Work out the finished part from the listing and answer in its coordinate system (mm). A direction names the side the tool comes from. Give positions to 0.01 mm unless a question says otherwise; leave off trailing zeros. Loops run counter-clockwise (first coordinate to the right, second up) from the corner with the lowest first, then second, coordinate; pieces in that order, holes last. Notation, with made-up numbers: (-17.75, 37.5) - (25.25, 37.5) arc R28 ccw to (25.25, 60.5) - close; hole circle Ø2 at (-1.5, -5). An arc over 180 degrees is marked (long way). One line per item, written item: value.
from build123d import *

# Parameters (mm, degrees)
SKETCH1_R           = 1.45
SKETCH1_W           = 3.4
SKETCH1_H           = 6.165
BOSS_EXTRUDE1_DEPTH = 6


with BuildPart() as part:
    # Sketch1 → Boss-Extrude1 (new body)
    with BuildSketch(Plane.XY):
        with BuildLine():
            Line((589.771388, 466.232899), (612.771388, 466.232899))
            ThreePointArc((612.771388, 466.232899), (618.521388, 460.482899), (612.771388, 454.732899))
            Line((612.771388, 454.732899), (589.771388, 454.732899))
            Line((589.771388, 454.732899), (586.771388, 454.732899))
            ThreePointArc((586.771388, 454.732899), (581.021388, 460.482899), (586.771388, 466.232899))
            Line((586.771388, 466.232899), (589.771388, 466.232899))
        make_face()
        with Locations((589.771388, 460.482899)):
            Circle(SKETCH1_R, mode=Mode.SUBTRACT)
        with Locations((612.771388, 460.482899)):
            Circle(SKETCH1_R, mode=Mode.SUBTRACT)
        with Locations((595.021388, 460.482899)):
            Rectangle(SKETCH1_W, SKETCH1_H, mode=Mode.SUBTRACT)
    extrude(amount=BOSS_EXTRUDE1_DEPTH)


solid = part.part
1. The mould has two halves that part along Y. Classify faces 3 (the flat face through (593.321, 460, 3)), 4 (the flat face through (600, 454.733, 3)), 5 (the flat face through (600, 461, 6)): released by +Y, released by -Y, zero draft, split by the parting line, or undercut.
Output:
face 3: undercut
face 4: released by -Y
face 5: zero draft
2. Section B-B (y = 461.25) is taken. Write down the section's boundary in (x, z).
Output:
outline: (581.07, 0) - (588.54, 0) - (588.54, 6) - (581.07, 6) - close; (591, 0) - (593.32, 0) - (593.32, 6) - (591, 6) - close; (596.72, 0) - (611.54, 0) - (611.54, 6) - (596.72, 6) - close; (614, 0) - (618.47, 0) - (618.47, 6) - (614, 6) - close
3. Section A-A (x = 595.5) is taken. Write down the section's boundary in (y, z), and give its area (3 significant figures).
Output:
outline: (454.73, 0) - (457.4, 0) - (457.4, 6) - (454.73, 6) - close; (463.57, 0) - (466.23, 0) - (466.23, 6) - (463.57, 6) - close
area: 32.0 mm²
4. Find the intervals of material crossed by line 1 along X through (y, z) = (459.5, 5.3); line 2 along X through (y, z) = (461, 4.15); line 3 along Y through (x, z) = (590, 5.7), in increasing order.
Output:
line 1: x = 581.11 to 588.71, 590.84 to 593.32, 596.72 to 611.71, 613.84 to 618.44
line 2: x = 581.04 to 588.42, 591.13 to 593.32, 596.72 to 611.42, 614.13 to 618.5
line 3: y = 454.73 to 459.05, 461.91 to 466.23
5. For faces 1 (the flat face through (595, 457.4, 3)), 2 (the flat face through (600, 466.233, 3)), determine the directions among +Z, -Z, +X, -X, +Y, -Y from which every point of the face is accessible in a straight line to the end or side of a thin tool.
Output:
face 1: +Z, -Z
face 2: +Z, -Z, +X, -X, +Y
6. Section D-D (x = 590) is taken. Write down the section's boundary in (y, z).
Output:
outline: (454.73, 0) - (459.05, 0) - (459.05, 6) - (454.73, 6) - close; (461.91, 0) - (466.23, 0) - (466.23, 6) - (461.91, 6) - close
7. Section C-C (z = 2) is taken. Write down the section's boundary in (x, y).
Output:
outline: (586.77, 454.73) - (612.77, 454.73) arc R5.75 ccw to (612.77, 466.23) - (586.77, 466.23) arc R5.75 ccw to start; hole circle Ø2.9 at (589.77, 460.48); hole (593.32, 457.4) - (596.72, 457.4) - (596.72, 463.57) - (593.32, 463.57) - close; hole circle Ø2.9 at (612.77, 460.48)
8. A flat-ended cylindrical pin translates along its axis: pin 1 Ø3 at (y, z) = (464.5, 1) entering from -X. Find the tip coordinate at first contact, or state that the pin passes through.
Output:
pin 1: stops at x = 581.6
